Part model, mm, in its own coordinate system. Give positions to 0.01 mm unless a question says otherwise; leave off trailing zeros. Write each loop counter-clockwise with the first axis right and the second up, starting at its lowest first coordinate (ties: lowest second). Pieces come first, ordered by that corner, then holes. Notation, with made-up numbers: (71.25, 15.25) - (115.25, 15.25) arc R34 cw to (115.25, 46.25) - close; hole circle Ø2 at (2.25, 50.5). An arc over 180 degrees is marked (long way). Answer as a JSON object with one key per item and string values. Group by question number.
```python
from build123d import *

# Parameters (mm, degrees)
SKETCH1_W               = 203.835
SKETCH1_H               = 38.1
BOSS_EXTRUDE1_DEPTH     = 2.54
SKETCH2_W               = 198.501
SKETCH2_H               = 2.54
BOSS_EXTRUDE2_DEPTH     = 5.08
CUT_EXTRUDE1_DEPTH      = 3.81
CUT_EXTRUDE1_DEPTH_BACK = 3.81
FILLET2_R               = 2.54


with BuildPart() as part:
    # Sketch1 → Boss-Extrude1 (new body)
    with BuildSketch(Plane(origin=(0, 0, 0), x_dir=(1, 0, 0), z_dir=(0, 1, 0))):
        Rectangle(SKETCH1_W, SKETCH1_H)
    extrude(amount=BOSS_EXTRUDE1_DEPTH)

    # Sketch2 → Boss-Extrude2 (add)
    with BuildSketch(Plane.XY.offset(19.05)):
        with Locations((0, 3.81)):
            Rectangle(SKETCH2_W, SKETCH2_H)
    extrude(amount=-BOSS_EXTRUDE2_DEPTH)

    # Sketch5 → Cut-Extrude1 (cut, two sides)
    with BuildSketch(Plane(origin=(0, 0, 0), x_dir=(0, 0, -1), z_dir=(1, 0, 0))) as cut_extrude1_sk:
        Polygon((16.51, 2.54), (12.7, 1.27), (8.89, 2.54), align=None)
    extrude(amount=CUT_EXTRUDE1_DEPTH, mode=Mode.SUBTRACT)
    extrude(cut_extrude1_sk.sketch, amount=-CUT_EXTRUDE1_DEPTH_BACK, mode=Mode.SUBTRACT)

    # Fillet2
    fillet2_edges = [part.edges().sort_by_distance(p)[0] for p in [
        (0, 1.27, -12.7),
    ]]
    fillet(fillet2_edges, radius=FILLET2_R)


solid = part.part
```
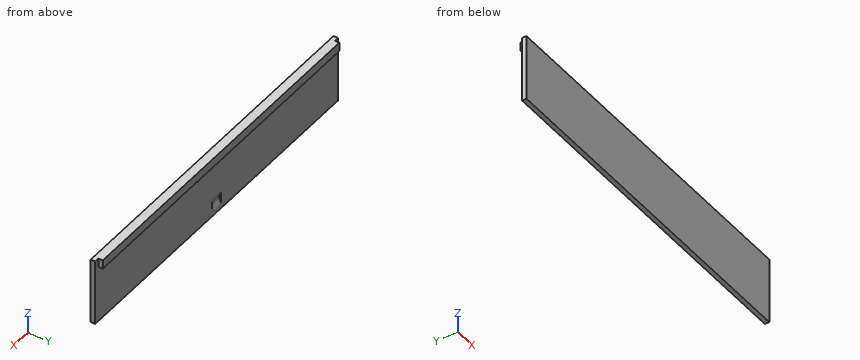
1) Drill centre lines: line 1 along Y through (x, z) = (65, -4.5); line 2 along Z through (x, y) = (-75.5, 4.6); line 3 along X through (y, z) = (3.75, 15.5). Where is each one in solid material? Low to high. Write a range as from..to.
2) Saw through at C-C (z = 6). List the corners of the cut face in (x, y), and give its area (3 significant figures).
3) Saw through at B-B (y = 3.55). List the corners of the cut face in (x, z).
4) Drop flat-ended pins along their axis: P1, Ø4, axis at x = -37.5, z = 7.5, coming from the +Y side; P2, Ø0.8, axis at y = 4, z = 17, coming from the -X side; P3, Ø1.3, axis at y = 4, z = 16, coming from the +X side; P4, Ø2, axis at y = 4.5, z = 5, coming from the -X side. Give the stop position or say it passes through.
5) Saw through at A-A (x = 16). List the corners of the cut face in (y, z), and give its area (3 significant figures).
Checks:
{
 "1": {"line 1": "0..2.54", "line 2": "13.97..19.05", "line 3": "-99.25..99.25"},
 "2": {"outline": "(-101.92, 0) - (101.92, 0) - (101.92, 2.54) - (-101.92, 2.54) - close", "area": "518 mm2"},
 "3": {"outline": "(-99.25, 13.97) - (99.25, 13.97) - (99.25, 19.05) - (-99.25, 19.05) - close"},
 "4": {"P1": "y = 2.54", "P2": "x = -99.25", "P3": "x = 99.25", "P4": "through"},
 "5": {"outline": "(0, -19.05) - (2.54, -19.05) - (2.54, 13.97) - (5.08, 13.97) - (5.08, 19.05) - (0, 19.05) - close", "area": "110 mm2"}
}
